Read the model definition and answer for the solid it produces. Units are mm, in the model's axes. Round coordinates to 2 decimals unless told otherwise and drop trailing zeros. Loops run counter-clockwise (first coordinate to the right, second up) from the corner with the lowest first, then second, coordinate; pieces in that order, holes last. Notation, with made-up numbers: (68, -9) -> (82, -9) arc R21 ccw to (82, 14) -> close; hole circle Ø2 at (-17, 3.25). An arc over 180 degrees is marked (long way). Put each result on its own line as item: value.
from build123d import *

# Parameters (mm, degrees)
F1_DEPTH = 9
F2_R     = 4.5
F3_DEPTH = 30
F5_W     = 100
F5_H     = 30
F6_DEPTH = 25


# Not quite as in the source:
# - the program builds the solid bodies; features that only make, move or delete a surface that nothing else refers to are left out


with BuildPart() as f1:
    # F0 (on Front) → F1 (new body)
    with BuildSketch(Plane.XZ):
        with BuildLine():
            Line((112.4640594495, 109.3449960649), (-84.5359405505, 109.3449960649))
            ThreePointArc((-84.5359405505, 109.3449960649), (-119.8912796099, 94.7003351242), (-134.5359405505, 59.3449960649))
            Line((-134.5359405505, 59.3449960649), (-134.5359405505, -50.6550039351))
            ThreePointArc((-134.5359405505, -50.6550039351), (-119.8912796099, -86.0103429944), (-84.5359405505, -100.6550039351))
            Line((-84.5359405505, -100.6550039351), (112.4640594495, -100.6550039351))
            ThreePointArc((112.4640594495, -100.6550039351), (147.8193985088, -86.0103429944), (162.4640594495, -50.6550039351))
            Line((162.4640594495, -50.6550039351), (162.4640594495, 59.3449960649))
            ThreePointArc((162.4640594495, 59.3449960649), (147.8193985088, 94.7003351242), (112.4640594495, 109.3449960649))
        make_face()
    extrude(amount=F1_DEPTH)

    # F2 (on face) → F3 (join)
    with BuildSketch(Plane.XZ.offset(9)):
        with Locations((-104.5359405505, 69.3449960649)):
            Circle(F2_R)
    extrude(amount=F3_DEPTH)

    # F5 (on face) → F6 (cut)
    with BuildSketch(Plane.XZ.offset(9)):
        with Locations((112.4640594495, 74.3449960649)):
            Rectangle(F5_W, F5_H)
    extrude(amount=-F6_DEPTH, mode=Mode.SUBTRACT)


solid = f1.part
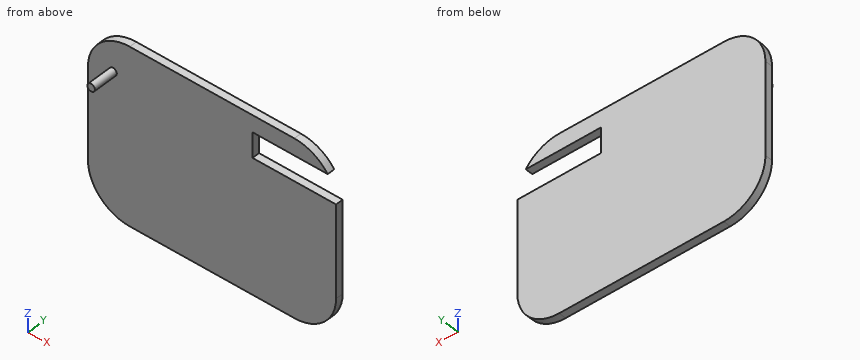
Item 1: The part is cut by section D-D (y = -18). Determine the outline of the cut face in (x, z) (3 decimals), then the cut area to 3 significant figures.
Derived:
outline: circle Ø9 at (-104.536, 69.345)
area: 63.6 mm^2
Item 2: Find the intervals of material crossed by line 1 along Y through (x, z) = (30.5, -22); line 2 along X through (y, z) = (-5, 73.5); line 3 along Z through (x, y) = (-102, -2), in increasing order.
Derived:
line 1: y = -9 to 0
line 2: x = -132.49 to 62.46
line 3: z = -97.51 to 106.2
Item 3: The part is cut by section A-A (x = 109.5). Determine the outline of the cut face in (y, z) (3 decimals).
Derived:
outline: (-9, -100.655) -> (0, -100.655) -> (0, 59.345) -> (-9, 59.345) -> close; (-9, 89.345) -> (0, 89.345) -> (0, 109.345) -> (-9, 109.345) -> close
Item 4: The part is cut by section C-C (z = 42.5). Determine the outline of the cut face in (x, y).
Derived:
outline: (-134.54, -9) -> (162.46, -9) -> (162.46, 0) -> (-134.54, 0) -> close
Item 5: The part is cut by section B-B (x = 53). Determine the outline of the cut face in (y, z) (3 decimals).
Derived:
outline: (-9, -100.655) -> (0, -100.655) -> (0, 109.345) -> (-9, 109.345) -> close
Item 6: Flat-ended cylindrical pins translate along their axes: pin 1 Ø3 at (x, z) = (-12.5, -11.5) entering from -Y; pin 2 Ø10 at (y, z) = (-3.5, 77.5) entering from +X; pin 3 Ø10 at (y, z) = (-13, 70) entering from -X. Find the tip coordinate at first contact, or state that the pin passes through.
Derived:
pin 1: stops at y = -9
pin 2: stops at x = 62.46
pin 3: stops at x = -133.95
